Build history of the part. All positions in model axes, mm. Give positions to 0.01 mm unless a question says otherwise; leave off trailing zeros. Order: outer loops, then holes, each group sorted by start corner. A loop starts at its lowest first (then second) coordinate and runs counter-clockwise, first axis right, second up. Notation, with made-up numbers: M 22,82 L 56,82 A23 cw 56,93 Z; hole C 88.5,66.25 d6. An arc over 180 degrees is marked long. One line per item, written item: value.
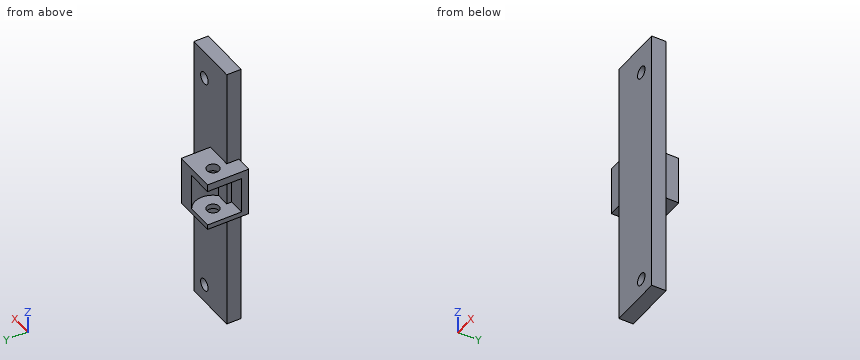
from build123d import *

# Parameters (mm, degrees)
BOSS_EXTRUDE1_DEPTH      = 21.59
SKETCH2_W                = 22.352
SKETCH2_H                = 21.59
SKETCH2_R                = 3.175
BOSS_EXTRUDE2_DEPTH      = 3.81
BOSS_EXTRUDE3_START      = -2.54
SKETCH3_R                = 3.175
BOSS_EXTRUDE3_DEPTH      = 2.54
BOSS_EXTRUDE4_DEPTH      = 1.164777
BOSS_EXTRUDE4_DEPTH_BACK = 6.35
SKETCH4_W                = 27.94
SKETCH4_H                = 142.24
SKETCH4_R                = 3.175


with BuildPart() as part:
    # Sketch1 → Boss-Extrude1 (new body)
    with BuildSketch(Plane.XY):
        with BuildLine():
            Line((801.338321143, 96.160777143), (792.583825879, 96.160777143))
            Line((792.583825879, 96.160777143), (792.583825879, 92.376177143))
            Line((792.583825879, 92.376177143), (814.935825879, 92.376177143))
            Line((814.935825879, 92.376177143), (814.935825879, 113.966177143))
            Line((814.935825879, 113.966177143), (806.045825879, 113.966177143))
            ThreePointArc((806.045825879, 113.966177143), (810.863321143, 105.685777143), (806.045825879, 97.405377143))
            ThreePointArc((806.045825879, 97.405377143), (803.772947911, 96.477182381), (801.338321143, 96.160777143))
        make_face()
    extrude(amount=-BOSS_EXTRUDE1_DEPTH)

    # Sketch2 → Boss-Extrude2 (add)
    with BuildSketch(Plane.XY):
        with Locations((803.759825879, 103.171177143)):
            Rectangle(SKETCH2_W, SKETCH2_H)
        with Locations((801.338321143, 105.685777143)):
            Circle(SKETCH2_R, mode=Mode.SUBTRACT)
    extrude(amount=BOSS_EXTRUDE2_DEPTH)

    # Sketch3 → Boss-Extrude3 (add)
    with BuildSketch(Plane(origin=(0, 0, -21.59), x_dir=(-1, 0, 0), z_dir=(0, 0, -1)).offset(BOSS_EXTRUDE3_START)):
        with BuildLine():
            Line((-801.338321143, 96.160777143), (-792.583825879, 96.160777143))
            Line((-792.583825879, 96.160777143), (-792.583825879, 113.966177143))
            Line((-792.583825879, 113.966177143), (-806.045825879, 113.966177143))
            ThreePointArc((-806.045825879, 113.966177143), (-810.546915906, 103.251150375), (-801.338321143, 96.160777143))
        make_face()
        with Locations(Location((-801.338321143, 105.685777143, 0), (0, 0, 180))):
            Circle(SKETCH3_R, mode=Mode.SUBTRACT)
    extrude(amount=BOSS_EXTRUDE3_DEPTH)

    # Sketch4 → Boss-Extrude4 (add, two sides: drawn at the far end of the back side and taken through both)
    with BuildSketch(Plane.XZ.offset(-92.376177143).offset(-BOSS_EXTRUDE4_DEPTH_BACK)):
        with Locations((814.935825879, -16.51)):
            Rectangle(SKETCH4_W, SKETCH4_H)
        with Locations(Location((820.039, 39.768571429, 0), (0, 0, 270))):
            Circle(SKETCH4_R, mode=Mode.SUBTRACT)
        with Locations(Location((820.039, -78.16, 0), (0, 0, 270))):
            Circle(SKETCH4_R, mode=Mode.SUBTRACT)
    extrude(amount=BOSS_EXTRUDE4_DEPTH + BOSS_EXTRUDE4_DEPTH_BACK)


solid = part.part
1) Pin check, flat tips, straight feed: pin 1 (1 mm diameter, centred on y = 95.5, z = -56.5, fed in from -X); pin 2 (5 mm diameter, centred on x = 810, y = 111, fed in from +Z); pin 3 (2 mm diameter, centred on x = 808, y = 107.5, fed in from -Z). Stop position of each tip, or through.
Check values:
pin 1: x = 800.97
pin 2: z = 3.81
pin 3: z = -21.59
2) Saw through at B-B, the plane z = -51.5. Write the cut outline in (x, y).
Check values:
outline: M 800.97,91.21 L 828.91,91.21 L 828.91,98.73 L 800.97,98.73 Z
3) Drill centre lines: probe 1 along Z at (x, y) = (806, 99); probe 2 along X at (y, z) = (95.5, -78.16); probe 3 along Y at (x, z) = (811, -65.5). Where is each one in solid material? Low to high. Write a range as from..to.
Check values:
probe 1: -21.59..-19.05, 0..3.81
probe 2: 800.97..816.86, 823.21..828.91
probe 3: 91.21..98.73
4) Saw through at A-A, the plane z = -78.16. Write the cut outline in (x, y), then the cut area to 3 significant figures.
Check values:
outline: M 800.97,91.21 L 816.86,91.21 L 816.86,98.73 L 800.97,98.73 Z; M 823.21,91.21 L 828.91,91.21 L 828.91,98.73 L 823.21,98.73 Z
area: 162 mm^2
